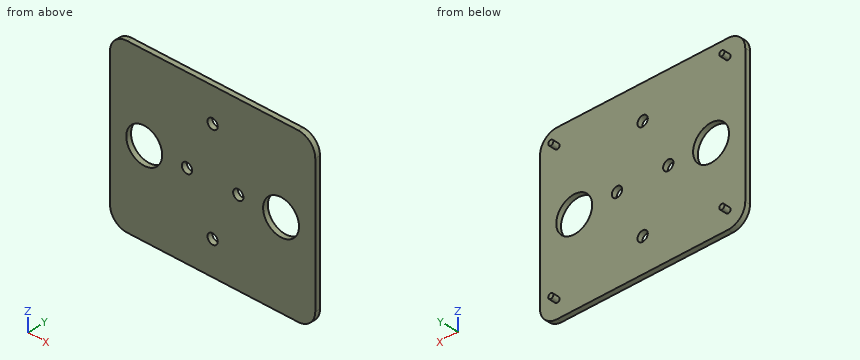
```python
from build123d import *

# Parameters (mm, degrees)
ESQUISSE1_W             = 120
ESQUISSE1_H             = 100
BOSS_EXTRU_1_DEPTH      = 3
CONG_1_R                = 10
ESQUISSE2_R             = 1.5
BOSS_EXTRU_2_DEPTH      = 4
ESQUISSE3_R             = 10.5
ESQUISSE3_R_2           = 3
ENL_V_MAT_EXTRU_1_DEPTH = 4


with BuildPart() as part:
    # Esquisse1 → Boss.-Extru.1 (new body)
    with BuildSketch(Plane(origin=(0, 0, 0), x_dir=(1, 0, 0), z_dir=(0, 1, 0))):
        with Locations((-60, 50)):
            Rectangle(ESQUISSE1_W, ESQUISSE1_H)
    extrude(amount=BOSS_EXTRU_1_DEPTH)

    # Congé1
    cong_1_edges = [part.edges().sort_by_distance(p)[0] for p in [
        (0, 1.5, 0),
        (-120, 1.5, 0),
        (-120, 1.5, -100),
        (0, 1.5, -100),
    ]]
    fillet(cong_1_edges, radius=CONG_1_R)

    # Esquisse2 → Boss.-Extru.2 (add)
    with BuildSketch(Plane(origin=(0, 3, 0), x_dir=(1, 0, 0), z_dir=(0, 1, 0))):
        with Locations((-110, 90)):
            Circle(ESQUISSE2_R)
        with Locations((-10, 90)):
            Circle(ESQUISSE2_R)
        with Locations((-10, 10)):
            Circle(ESQUISSE2_R)
        with Locations((-110, 10)):
            Circle(ESQUISSE2_R)
    extrude(amount=BOSS_EXTRU_2_DEPTH)

    # Esquisse3 → Enlèv. mat.-Extru.1 (cut, through all)
    with BuildSketch(Plane(origin=(0, 3, 0), x_dir=(1, 0, 0), z_dir=(0, 1, 0))):
        with Locations((-100, 50)):
            Circle(ESQUISSE3_R)
        with Locations((-20, 50)):
            Circle(ESQUISSE3_R)
        with Locations((-75, 50)):
            Circle(ESQUISSE3_R_2)
        with Locations((-45, 50)):
            Circle(ESQUISSE3_R_2)
        with Locations((-60, 80)):
            Circle(ESQUISSE3_R_2)
        with Locations((-60, 20)):
            Circle(ESQUISSE3_R_2)
    extrude(amount=-ENL_V_MAT_EXTRU_1_DEPTH, mode=Mode.SUBTRACT)


solid = part.part
```
CAD build for the part. Positions are in the model's coordinates, mm. Give positions to 0.01 mm unless a question says otherwise; leave off trailing zeros. Order: outer loops, then holes, each group sorted by start corner. A loop starts at its lowest first (then second) coordinate and runs counter-clockwise, first axis right, second up. Notation, with made-up numbers: M -25.75,42.25 L -14.75,42.25 A33 cw -14.75,77.25 Z; hole C 17,18 d11. An arc over 180 degrees is marked long. Put each result on its own line as item: value. Start each with the question number.
(1) Saw through at D-D, the plane y = 1.75. Write the cut outline in (x, z), then the cut area to 3 significant figures.
(2) Saw through at C-C, the plane x = -60. Write the cut outline in (y, z).
(3) Flat gauge pins, fed straight in: pin 1 Ø7 at (x, z) = (-60, -80) entering from +Y; pin 2 Ø19 at (x, z) = (-20, -50) entering from +Y; pin 3 Ø2 at (y, z) = (6, -88) entering from +X. Where does each tip first touch, or does it go through?
(4) Saw through at A-A, the plane z = -50. Write the cut outline in (x, y), then the cut area to 3 significant figures.
(5) Saw through at B-B, the plane x = -100. Write the cut outline in (y, z).
(6) Drill centre lines: line 1 along X through (y, z) = (1.2, -50); line 2 along Z through (x, y) = (-100, 1.6); line 3 along X through (y, z) = (1.5, -52). Where is each one in solid material? Low to high.
Check result:
1. outline: M -120,-90 A10 ccw -110,-100 L -10,-100 A10 ccw 0,-90 L 0,-10 A10 ccw -10,0 L -110,0 A10 ccw -120,-10 Z; hole C -100,-50 d21; hole C -75,-50 d6; hole C -60,-80 d6; hole C -60,-20 d6; hole C -45,-50 d6; hole C -20,-50 d21
1. area: 11,100 mm2
2. outline: M 0,-100 L 3,-100 L 3,-83 L 0,-83 Z; M 0,-77 L 3,-77 L 3,-23 L 0,-23 Z; M 0,-17 L 3,-17 L 3,0 L 0,0 Z
3. pin 1: stops at y = 3
3. pin 2: passes through
3. pin 3: stops at x = -8.88
4. outline: M -120,0 L -110.5,0 L -110.5,3 L -120,3 Z; M -89.5,0 L -78,0 L -78,3 L -89.5,3 Z; M -72,0 L -48,0 L -48,3 L -72,3 Z; M -42,0 L -30.5,0 L -30.5,3 L -42,3 Z; M -9.5,0 L 0,0 L 0,3 L -9.5,3 Z
4. area: 198 mm2
5. outline: M 0,-100 L 3,-100 L 3,-60.5 L 0,-60.5 Z; M 0,-39.5 L 3,-39.5 L 3,0 L 0,0 Z
6. line 1: x = -120 to -110.5, -89.5 to -78, -72 to -48, -42 to -30.5, -9.5 to 0
6. line 2: z = -100 to -60.5, -39.5 to 0
6. line 3: x = -120 to -110.31, -89.69 to -77.24, -72.76 to -47.24, -42.76 to -30.31, -9.69 to 0
